Check sheet for the modelled part. Datum: model origin and axes. Units: mm. Coordinates: 2 decimals unless noted, no trailing zeros. Write each loop counter-clockwise with the first axis right and the second up, starting at its lowest first coordinate (ties: lowest second). Pieces come first, ordered by that corner, then holes. Notation, with made-up numbers: M 37.25,51.25 L 78.25,51.25 A21 ccw 78.25,76.25 Z; hole C 38.25,-12.75 d2. An arc over 180 degrees is marked long. Answer as CSV lines item,"result". Start each with the question number.
1) Section check A-A (x = 88.9). Record the cut outline in (y, z), and give its area (3 significant figures).
2) Material ranges on L1, parallel to Z at x = -88.9, y = 0.75; L2, parallel to Z at x = 91, y = 0.25, recorded low to high. Write a range as [from, to].
3) Section check B-B (z = 0). Record the cut outline in (x, y).
from build123d import *

# Parameters (mm, degrees)
F0_W     = 228.6
F0_H     = 25.4
F0_R     = 3.81
F0_R_2   = 2.54
F1_DEPTH = 12.7


with BuildPart() as f1:
    # F0 (on Front) → F1 (new body, symmetric)
    with BuildSketch(Plane.XZ):
        Rectangle(F0_W, F0_H)
        with Locations((-88.9, 0)):
            Circle(F0_R, mode=Mode.SUBTRACT)
        with Locations((88.9, 0)):
            Circle(F0_R, mode=Mode.SUBTRACT)
        with Locations((88.9, 0)):
            Circle(F0_R)
        with Locations((88.9, 0)):
            Circle(F0_R_2, mode=Mode.SUBTRACT)
        with Locations((-88.9, 0)):
            Circle(F0_R)
        with Locations((-88.9, 0)):
            Circle(F0_R_2, mode=Mode.SUBTRACT)
    extrude(amount=F1_DEPTH, both=True)


solid = f1.part
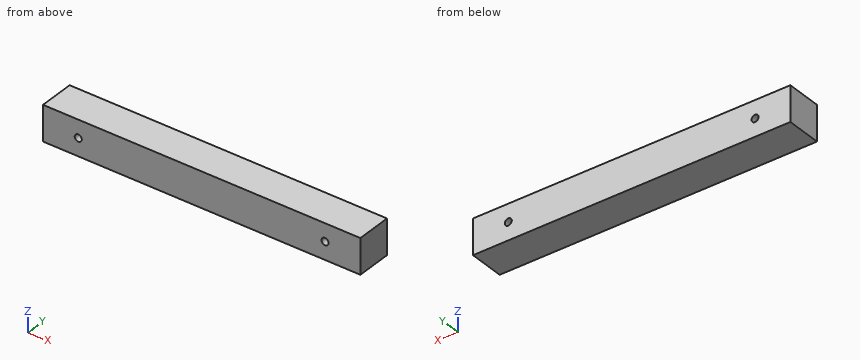
Results found:
1,outline,"M -12.7,-12.7 L 12.7,-12.7 L 12.7,-2.54 L -12.7,-2.54 Z; M -12.7,2.54 L 12.7,2.54 L 12.7,12.7 L -12.7,12.7 Z"
1,area,"516 mm2"
2,L1,"z = [-12.7, -2.54], [2.54, 12.7]"
2,L2,"z = [-12.7, -1.43], [1.43, 12.7]"
3,outline,"M -114.3,-12.7 L -91.44,-12.7 L -91.44,12.7 L -114.3,12.7 Z; M -86.36,-12.7 L 86.36,-12.7 L 86.36,12.7 L -86.36,12.7 Z; M 91.44,-12.7 L 114.3,-12.7 L 114.3,12.7 L 91.44,12.7 Z"
